The model under review builds one solid part; all positions refer to its coordinate system, in mm. Give positions to 0.01 mm unless a question says otherwise; leave off trailing zeros. Loops run counter-clockwise (first coordinate to the right, second up) from the corner with the lowest first, then second, coordinate; pieces in that order, holes last. Notation, with made-up numbers: (-1, -18.75) -> (35, -18.75) arc R27 cw to (35, 9.25) -> close; hole circle Ø1 at (-27.5, -13). An arc over 180 degrees is marked (long way). Write each question's results on one line, items separated by ' | '. Start each with the question number.
Q1. Wall thickness on L1, parallel to Y at x = -176.5, z = -19; L2, parallel to Z at x = 551, y = 35; L3, parallel to Y at x = -233, z = -3: over which ranges is each line inside the solid? List them lowest first. Write a range as [from, to].
Q2. Insertion check: pin 1 Ø1.5 at (y, z) = (8, -59.5) entering from +X; pin 2 Ø3 at (x, y) = (-241.5, 21.5) entering from -Z; pin 3 Ø1.9 at (x, z) = (192.5, -4.5) entering from +Y; pin 4 Ø8 at (x, z) = (-204, -41) entering from +Y. Each pin has a flat end and moves straight along its axis. Give the tip position at first contact, or say it passes through.
Q3. We need section C-C (z = -28). Write out the cut boundary in (x, y), plus the area to 3 significant figures.
Q4. We need section A-A (x = -661.5). Write out the cut boundary in (y, z), plus the area to 3 significant figures.
Q5. We need section B-B (x = 447.5). Write out the cut boundary in (y, z).
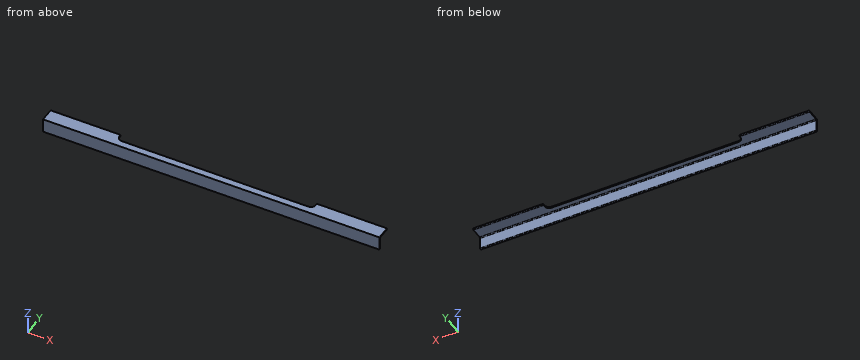
from build123d import *

# Parameters (mm, degrees)
BOSS_EXTRUDE1_DEPTH      = 914.4
BOSS_EXTRUDE1_DEPTH_BACK = 914.4
SKETCH2_W                = 1066.8
SKETCH2_H                = 38.1
CUT_EXTRUDE1_DEPTH       = 77.2
FILLET1_R                = 25.4


with BuildPart() as part:
    # Sketch1 → Boss-Extrude1 (new body, two sides)
    with BuildSketch(Plane(origin=(0, 0, 0), x_dir=(0, 0, -1), z_dir=(1, 0, 0))) as boss_extrude1_sk:
        with BuildLine():
            Line((0, 76.2), (0, 0))
            Line((0, 0), (76.2, 0))
            Line((76.2, 0), (76.2, 1.27))
            ThreePointArc((76.2, 1.27), (74.712102448, 4.862102448), (71.12, 6.35))
            Line((71.12, 6.35), (11.43, 6.35))
            ThreePointArc((11.43, 6.35), (7.837897552, 7.837897552), (6.35, 11.43))
            Line((6.35, 11.43), (6.35, 71.12))
            ThreePointArc((6.35, 71.12), (4.862102448, 74.712102448), (1.27, 76.2))
            Line((1.27, 76.2), (0, 76.2))
        make_face()
    extrude(amount=BOSS_EXTRUDE1_DEPTH)
    extrude(boss_extrude1_sk.sketch, amount=-BOSS_EXTRUDE1_DEPTH_BACK)

    # Sketch2 → Cut-Extrude1 (cut, through all)
    with BuildSketch(Plane.XY):
        with Locations((0, 57.15)):
            Rectangle(SKETCH2_W, SKETCH2_H)
    extrude(amount=-CUT_EXTRUDE1_DEPTH, mode=Mode.SUBTRACT)

    # Fillet1
    fillet1_edges = [part.edges().sort_by_distance(p)[0] for p in [
        (-533.4, 38.1, -3.175),
        (533.4, 38.1, -3.175),
    ]]
    fillet(fillet1_edges, radius=FILLET1_R)


solid = part.part
Output:
1) L1: [0, 6.35] | L2: [-6.35, 0] | L3: [0, 38.1]
2) pin 1: through | pin 2: z = -6.35 | pin 3: y = 38.1 | pin 4: y = 6.35
3) outline: (-914.4, 0) -> (914.4, 0) -> (914.4, 6.35) -> (-914.4, 6.35) -> close | area: 11,600 mm2
4) outline: (0, -76.2) -> (1.27, -76.2) arc R5.08 ccw to (6.35, -71.12) -> (6.35, -11.43) arc R5.08 cw to (11.43, -6.35) -> (71.12, -6.35) arc R5.08 ccw to (76.2, -1.27) -> (76.2, 0) -> (0, 0) -> close | area: 922 mm2
5) outline: (0, -76.2) -> (1.27, -76.2) arc R5.08 ccw to (6.35, -71.12) -> (6.35, -11.43) arc R5.08 cw to (11.43, -6.35) -> (38.1, -6.35) -> (38.1, 0) -> (0, 0) -> close
